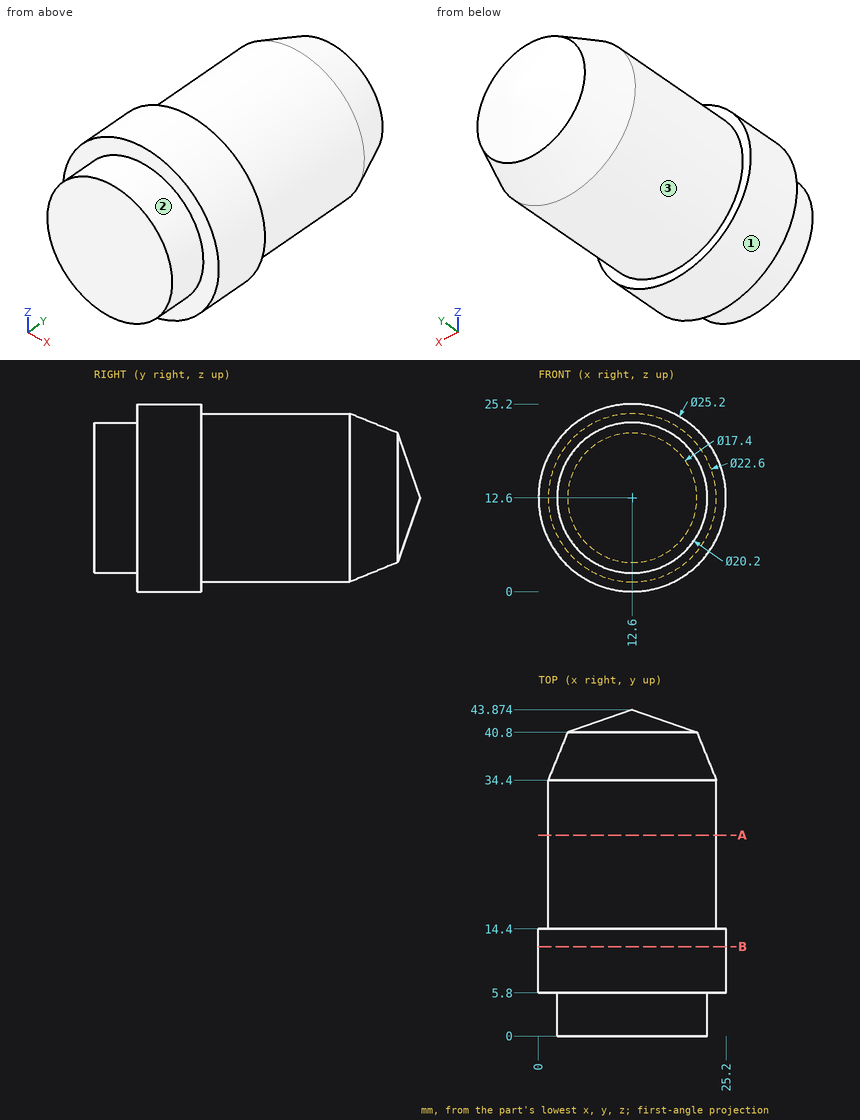
Verification items for this drawing (mm, ordinates from the low corner). A direction names the side the tool comes from. Coordinates: 2 decimals unless noted, no trailing zeros. Write each loop counter-clockwise with the first axis right and the second up, starting at its lowest first coordinate (ties: lowest second). Pieces come first, ordered by that corner, then holes. Notation, with made-up numbers: M -15.5,-19 L 18.5,-19 A27 ccw 18.5,5 Z; hole C 89,-20.5 d4. An arc over 180 degrees is marked long. Answer as a JSON object with one key per item and string values. Group by question number.
(1) Cross-section at A-A, the plane y = 27. Record the cut outline in (x, z).
(2) Tool access check on the marked faces 1, 2 and 3. Record the directions out of +Z, -Z, +X, -X, +Y, -Y that give a thin tool (end or side, any length) a straight path to the whole face; none if there is none.
(3) Cross-section at B-B, the plane y = 12. Record the cut outline in (x, z).
(4) Material ranges on line 1 (Y direction, x = 9, z = 24.25); line 2 (Y direction, x = 3.5, z = 16.75) (1 decimal); line 3 (X direction, y = 11.5, z = 3.5) (1 decimal), recorded low to high.
(5) Gauge pin test, flat ends, axial feed: pin 1 (3 mm diameter, centred on y = 31.5, z = 15, fed in from +X); pin 2 (10 mm diameter, centred on x = 9.5, z = 6, fed in from -Y); pin 3 (5 mm diameter, centred on x = 15, z = 11, fed in from +Y); pin 4 (1.5 mm diameter, centred on y = 17, z = 5.5, fed in from -X). Record the tip position at first contact, or that the pin passes through.
Reply:
{
 "1": {"outline": "C 12.6,12.6 d22.6"},
 "2": {"face 1": "+Y, -Y", "face 2": "-Y", "face 3": "+Y"},
 "3": {"outline": "C 12.6,12.6 d25.2"},
 "4": {"line 1": "5.8 to 14.4", "line 2": "0 to 37.6", "line 3": "3.9 to 21.3"},
 "5": {"pin 1": "x = 23.86", "pin 2": "y = 0", "pin 3": "y = 43.74", "pin 4": "x = 3.25"}
}
